The model under review builds one solid part; all positions refer to its coordinate system, in mm. A direction names the side the tool comes from. Round coordinates to 2 decimals unless told otherwise and drop trailing zeros. Write each loop counter-clockwise with the first axis right and the second up, starting at its lowest first coordinate (ties: lowest second). Pieces come first, ordered by that corner, then holes. Notation, with made-up numbers: (88, -19.75) -> (106, -19.75) arc R15 cw to (106, -14.75) -> close; hole circle Ø5 at (-16.5, 74.25). An arc over 180 degrees is marked (long way). Answer as a JSON object with one key per item and string values. Group by question number.
1) We need section A-A, the plane z = 114.5. Write out the cut boundary in (x, y).
2) We need section B-B, the plane x = -8.5. Write out the cut boundary in (y, z).
3) To check wall thickness, follow probe 1 along Y at (x, z) = (25, 222); probe 2 along Y at (x, z) = (21.5, 121); probe 3 along X at (y, z) = (4.75, 412.5). State the ranges of each line that lie inside material, in increasing order. Write a range as [from, to].
4) We need section C-C, the plane x = 10. Write out the cut boundary in (y, z).
5) Machinability: for faces 1 (the flat face through (0, -7, 30)), 2 (the flat face through (0, -6, 241)), which of the approach directions +Z, -Z, +X, -X, +Y, -Y give a long, thin tool a straight path to every point of the face, cutting with its end or side? Answer none if there is none.
6) Insertion check: pin 1 Ø8 at (x, y) = (-25, -2.5) entering from -Z. The pin has a flat end and moves straight along its axis. Give the tip position at first contact, or say it passes through.
from build123d import *

# Parameters (mm, degrees)
SKETCH_1_W               = 60
SKETCH_1_H               = 15
EXTRUDE_1_DEPTH          = 510
SKETCH_2_R               = 3
CUT_EXTRUDE_1_DEPTH      = 511.936639908
CUT_EXTRUDE_2_DEPTH      = 511.936639908
SKETCH_4_W               = 36.3
SKETCH_4_H               = 7
CUT_EXTRUDE_3_DEPTH      = 511.936639908
FILLET_1_R               = 2
CUT_EXTRUDE_4_DEPTH      = 512.101751122
CUT_EXTRUDE_6_DEPTH      = 512.101751122
CUT_EXTRUDE_6_DEPTH_BACK = 512.101751122
SKETCH_7_W               = 30
SKETCH_7_H               = 30


with BuildPart() as part:
    # 스케치1 → 보스-돌출1 (new body)
    with BuildSketch(Plane.XY):
        Rectangle(SKETCH_1_W, SKETCH_1_H)
    extrude(amount=EXTRUDE_1_DEPTH)

    # 스케치2 → 컷-돌출1 (cut, through all)
    with BuildSketch(Plane(origin=(0, 0, 0), x_dir=(-1, 0, 0), z_dir=(0, 0, -1))):
        with Locations((-25, -2.5)):
            Circle(SKETCH_2_R)
        with Locations((25, -2.5)):
            Circle(SKETCH_2_R)
    extrude(amount=-CUT_EXTRUDE_1_DEPTH, mode=Mode.SUBTRACT)

    # 스케치3 → 컷-돌출2 (cut, through all)
    with BuildSketch(Plane(origin=(0, 0, 0), x_dir=(-1, 0, 0), z_dir=(0, 0, -1))):
        with BuildLine():
            Line((-22.171572875, -6), (22.171572875, -6))
            ThreePointArc((22.171572875, -6), (20.939339828, -4.439339828), (20.5, -2.5))
            Line((20.5, -2.5), (25, -2.5))
            Line((25, -2.5), (25, 0.5))
            Line((25, 0.5), (-25, 0.5))
            Line((-25, 0.5), (-25, -2.5))
            Line((-25, -2.5), (-20.5, -2.5))
            ThreePointArc((-20.5, -2.5), (-20.939339828, -4.439339828), (-22.171572875, -6))
        make_face()
    extrude(amount=-CUT_EXTRUDE_2_DEPTH, mode=Mode.SUBTRACT)

    # 스케치4 → 컷-돌출3 (cut, through all)
    with BuildSketch(Plane(origin=(0, 0, 0), x_dir=(-1, 0, 0), z_dir=(0, 0, -1))):
        with Locations((0.006888359, 4)):
            Rectangle(SKETCH_4_W, SKETCH_4_H)
    extrude(amount=-CUT_EXTRUDE_3_DEPTH, mode=Mode.SUBTRACT)

    # 필렛1
    fillet_1_edges = [part.edges().sort_by_distance(p)[0] for p in [
        (-18.156888359, 0.5, 255),
        (18.143111641, 0.5, 255),
    ]]
    fillet(fillet_1_edges, radius=FILLET_1_R)

    # 스케치5 → 컷-돌출4 (cut, through all)
    with BuildSketch(Plane.XZ.offset(7.5)):
        Polygon((-30, 510), (-30, 450), (30, 510), align=None)
        Polygon((-30, 0), (30, 0), (-30, 60), align=None)
    extrude(amount=-CUT_EXTRUDE_4_DEPTH, mode=Mode.SUBTRACT)

    # 스케치7 → 컷-돌출6 (cut, two sides: drawn at the far end of the back side and taken through both)
    with BuildSketch(Plane.XZ.offset(7.5).offset(-CUT_EXTRUDE_6_DEPTH_BACK)):
        with Locations((15, 495)):
            Rectangle(SKETCH_7_W, SKETCH_7_H)
    extrude(amount=CUT_EXTRUDE_6_DEPTH + CUT_EXTRUDE_6_DEPTH_BACK, mode=Mode.SUBTRACT)


solid = part.part
Here are the results:
{
 "1": {"outline": "(-30, -7.5) -> (30, -7.5) -> (30, 7.5) -> (18.14, 7.5) -> (18.14, 2.5) arc R2 ccw to (20.14, 0.5) -> (25, 0.5) arc R3 cw (long way) to (22, -2.5) -> (20.5, -2.5) arc R4.5 ccw to (22.17, -6) -> (-22.17, -6) arc R4.5 ccw to (-20.5, -2.5) -> (-22, -2.5) arc R3 cw (long way) to (-25, 0.5) -> (-20.16, 0.5) arc R2 ccw to (-18.16, 2.5) -> (-18.16, 7.5) -> (-30, 7.5) -> close"},
 "2": {"outline": "(-7.5, 38.5) -> (-6, 38.5) -> (-6, 471.5) -> (-7.5, 471.5) -> close"},
 "3": {"probe 1": "y = [-7.5, -5.5], [0.5, 7.5]", "probe 2": "y = [-7.5, -6], [-5.33, -2.5], [0.5, 7.5]", "probe 3": "x = [-30, -18.16], [18.14, 30]"},
 "4": {"outline": "(-7.5, 20) -> (-6, 20) -> (-6, 480) -> (-7.5, 480) -> close"},
 "5": {"face 1": "-Z, -X, +Y, -Y", "face 2": "+Z, -Z"},
 "6": {"pin 1": "stops at z = 51"}
}
